from build123d import *

# Parameters (mm, degrees)
EXTRUDE_1_DEPTH     = 2
SKETCH_2_W          = 16
SKETCH_2_H          = 2
EXTRUDE_2_DEPTH     = 10
EXTRUDE_3_DEPTH     = 2
SKETCH_4_R          = 2.5
CUT_EXTRUDE_1_DEPTH = 3
SKETCH_5_R          = 2.5
CUT_EXTRUDE_2_DEPTH = 3


with BuildPart() as part:
    # 草图1 → 凸台-拉伸1 (new body)
    with BuildSketch(Plane(origin=(0, 0, 0), x_dir=(1, 0, 0), z_dir=(0, 1, 0))):
        with BuildLine():
            Line((8, 1.423853667), (-8, 1.423853667))
            Line((-8, 1.423853667), (-8, 13.423853667))
            ThreePointArc((-8, 13.423853667), (0, 21.423853667), (8, 13.423853667))
            Line((8, 13.423853667), (8, 1.423853667))
        make_face()
    extrude(amount=EXTRUDE_1_DEPTH)

    # 草图2 → 凸台-拉伸2 (add)
    with BuildSketch(Plane(origin=(0, 2, 0), x_dir=(1, 0, 0), z_dir=(0, 1, 0))):
        with Locations((0, 2.423853667)):
            Rectangle(SKETCH_2_W, SKETCH_2_H)
    extrude(amount=EXTRUDE_2_DEPTH)

    # 草图3 → 凸台-拉伸3 (add)
    with BuildSketch(Plane(origin=(0, 0, -3.423853667), x_dir=(-1, 0, 0), z_dir=(0, 0, -1))):
        with BuildLine():
            Line((-8, 12), (8, 12))
            ThreePointArc((8, 12), (0, 20), (-8, 12))
        make_face()
    extrude(amount=-EXTRUDE_3_DEPTH)

    # 草图4 → 切除-拉伸1 (cut, through all)
    with BuildSketch(Plane(origin=(0, 2, 0), x_dir=(1, 0, 0), z_dir=(0, 1, 0))):
        with Locations((0, 14.423853667)):
            Circle(SKETCH_4_R)
    extrude(amount=-CUT_EXTRUDE_1_DEPTH, mode=Mode.SUBTRACT)

    # 草图5 → 切除-拉伸2 (cut, through all)
    with BuildSketch(Plane(origin=(0, 0, -3.423853667), x_dir=(-1, 0, 0), z_dir=(0, 0, -1))):
        with Locations((0, 13)):
            Circle(SKETCH_5_R)
    extrude(amount=-CUT_EXTRUDE_2_DEPTH, mode=Mode.SUBTRACT)


solid = part.part
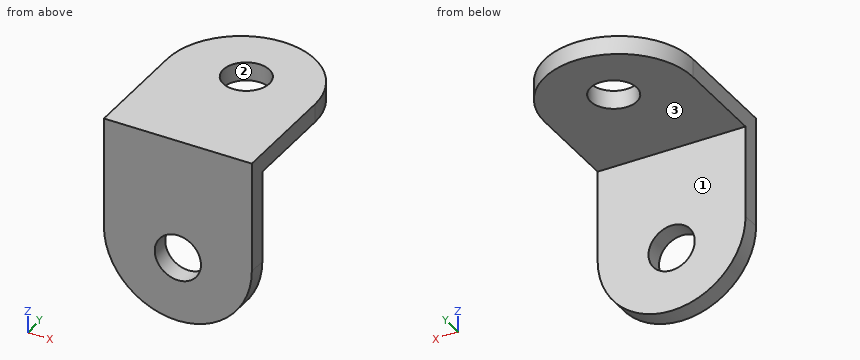
The listing builds one solid part. Answer for the finished solid, in the listing's coordinates (mm). Face numbers are marked on the shaded views. Round coordinates to 2 decimals unless told otherwise and drop trailing zeros. Order: outer loops, then holes, each group sorted by start corner. A loop starts at its lowest first (then second) coordinate and runs counter-clockwise, first axis right, second up. Notation, with made-up numbers: (-11.75, 1) -> (1.25, 1) arc R23 ccw to (1.25, 27) -> close; hole circle Ø9 at (-22.5, 27.25). An arc over 180 degrees is marked (long way). Put each result on its own line as item: value.
Q1. Determine the mould class of the marked faces 1, 2 and 3 for opening direction Y: pulls with the +Y half, pulls with the -Y half, needs draft (parallel to the pull), parting line crosses it, or undercut.
Results list:
face 1: pulls with the +Y half
face 2: undercut
face 3: needs draft
Q2. Consider line 1 along Y through (x, z) = (0, -2.55); line 2 along Z through (x, y) = (7.25, 2.25); line 3 along Y through (x, z) = (-5.25, -5.75). Determine where each line is inside the solid, lowest interval first.
Results list:
line 1: 0 to 10.5, 15.5 to 20
line 2: -3.42 to -1.42
line 3: 0 to 2
Q3. Section C-C, the plane z = -9.75 is taken. Write down the section's boundary in (x, y), and give its area (3 significant figures).
Results list:
outline: (-8, 0) -> (8, 0) -> (8, 2) -> (-8, 2) -> close
area: 32.0 mm^2
Q4. Section D-D, the plane x = -5.25 is taken. Write down the section's boundary in (y, z).
Results list:
outline: (0, -19.46) -> (2, -19.46) -> (2, -3.42) -> (18.04, -3.42) -> (18.04, -1.42) -> (0, -1.42) -> close
Q5. Each of these flat-tipped pins is pushed along its axis until it touches: P1, Ø8, axis at x = 0, z = -14.42, coming from the -Y side; P2, Ø4, axis at x = -0.5, z = -17.5, coming from the +Y side. Where does it stop, or does it pass through?
Results list:
P1: y = 0
P2: y = 2
Q6. Section A-A, the plane x = 0 is taken. Write down the section's boundary in (y, z).
Results list:
outline: (0, -21.42) -> (2, -21.42) -> (2, -16.92) -> (0, -16.92) -> close; (0, -11.92) -> (2, -11.92) -> (2, -3.42) -> (10.5, -3.42) -> (10.5, -1.42) -> (0, -1.42) -> close; (15.5, -3.42) -> (20, -3.42) -> (20, -1.42) -> (15.5, -1.42) -> close
Q7. Section B-B, the plane y = 13 is taken. Write down the section's boundary in (x, z), and give its area (3 significant figures).
Results list:
outline: (-7.94, -3.42) -> (-2.5, -3.42) -> (-2.5, -1.42) -> (-7.94, -1.42) -> close; (2.5, -3.42) -> (7.94, -3.42) -> (7.94, -1.42) -> (2.5, -1.42) -> close
area: 21.7 mm^2
